Could you check a few things on this model? Use its own coordinates, in mm. Face numbers are marked on the shaded views. A direction names the side the tool comes from. Coordinates: 2 decimals unless noted, no trailing zeros. Order: outer loops, then holes, each group sorted by start corner. A loop starts at its lowest first (then second) coordinate and runs counter-clockwise, first axis right, second up.
```python
from build123d import *

# Parameters (mm, degrees)
F0_W     = 76.2
F0_H     = 36.11469
F1_DEPTH = 58.42
F0_R     = 12.858175
F2_DEPTH = 25.4
F3_R     = 6.059169
F4_DEPTH = 76.2
F5_DEPTH = 76.2
F7_DEPTH = 38.1


with BuildPart() as f1:
    # F0 (on Top) → F1 (new body)
    with BuildSketch(Plane.XY):
        Rectangle(F0_W, F0_H)
    extrude(amount=F1_DEPTH)

    # F0 (on Top) → F2 (join)
    with BuildSketch(Plane.XY):
        with BuildLine():
            Line((72.961012, 28.850658), (-72.961012, 28.850658))
            ThreePointArc((-72.961012, 28.850658), (-101.81167, 0), (-72.961012, -28.850658))
            Line((-72.961012, -28.850658), (72.961012, -28.850658))
            ThreePointArc((72.961012, -28.850658), (101.81167, 0), (72.961012, 28.850658))
        make_face()
        with Locations((-72.961012, 0)):
            Circle(F0_R, mode=Mode.SUBTRACT)
        Rectangle(F0_W, F0_H, mode=Mode.SUBTRACT)
        with Locations((72.961012, 0)):
            Circle(F0_R, mode=Mode.SUBTRACT)
    extrude(amount=F2_DEPTH)

    # F3 (on face) → F4 (join)
    with BuildSketch(Plane(origin=(-38.1, 0, 0), x_dir=(0, -1, 0), z_dir=(-1, 0, 0))):
        with Locations((0, 58.42)):
            Circle(F3_R)
        with BuildLine():
            Line((6.059169, 58.42), (18.057345, 58.42))
            ThreePointArc((18.057345, 58.42), (0, 76.477345), (-18.057345, 58.42))
            Line((-18.057345, 58.42), (-6.059169, 58.42))
            ThreePointArc((-6.059169, 58.42), (0, 64.479169), (6.059169, 58.42))
        make_face()
    extrude(amount=-F4_DEPTH)

    # F3 (on face) → F5 (cut)
    with BuildSketch(Plane(origin=(-38.1, 0, 0), x_dir=(0, -1, 0), z_dir=(-1, 0, 0))):
        with Locations((0, 58.42)):
            Circle(F3_R)
    extrude(amount=-F5_DEPTH, mode=Mode.SUBTRACT)

    # F6 (on Front) → F7 (cut, symmetric)
    with BuildSketch(Plane.XZ):
        with BuildLine():
            Line((16.832678, 103.529039), (-16.832678, 103.529039))
            Line((-16.832678, 103.529039), (-16.832678, 48.142973))
            ThreePointArc((-16.832678, 48.142973), (0, 31.310296), (16.832678, 48.142973))
            Line((16.832678, 48.142973), (16.832678, 103.529039))
        make_face()
    extrude(amount=F7_DEPTH, both=True, mode=Mode.SUBTRACT)


solid = f1.part
```
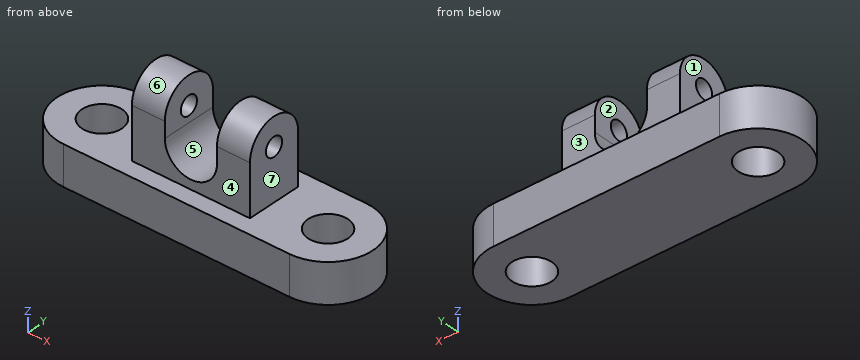
Item 1: Which directions (+Z, -Z, +X, -X, +Y, -Y) give clear straight access to the entire face, cutting with the end or side of a thin tool? Please do the marked faces 1, 2, 3 and 4.
Item 2: Thinking about a two-plate mould opening in X: for the marked faces 5, 6 and 7, which applies, +X half, -X half, draft (parallel to the pull), parting line (faces both ways), or undercut?
Item 3: I need wall thicknesses on line 1 (X direction, y = 1, z = 4.5); line 2 (Z direction, x = 33, y = 0); line 3 (X direction, y = 15.5, z = 56). Which ranges of each line are inside material? Lowest first, please.
Item 4: For pin 1 Ø18 at (y, z) = (-6, 44.5) entering from +X; pin 2 Ø4 at (x, y) = (-29, -17) entering from +Z; pin 3 Ø1.5 at (x, y) = (41, -22.5) entering from +Z, each with a flat end and sliding along its axis, tell me the tip position at first contact or that it passes through.
Item 5: Suppose I cut it at B-B (x = 33.5). List the corners of the cut face in (y, z) for me, and give its area (3 significant figures).
Item 6: Suppose I cut it at C-C (z = 36). List the corners of the cut face in (x, y) for me, and give its area (3 significant figures).
Item 7: Suppose I cut it at A-A (y = 0). List the corners of the cut face in (x, z) for me, and give its area (3 significant figures).
Item 8: Suppose I cut it at D-D (y = -9). List the corners of the cut face in (x, z) for me, and give its area (3 significant figures).
Geometry results:
1. face 1: +Z, -X, +Y, -Y
1. face 2: +Z, +Y, -Y
1. face 3: +Z, +X, -X, +Y
1. face 4: +Z, +X, -X, -Y
2. face 5: undercut
2. face 6: draft
2. face 7: +X half
3. line 1: x = -101.79 to -85.78, -60.14 to 60.14, 85.78 to 101.79
3. line 2: z = 0 to 52.36, 64.48 to 76.48
3. line 3: x = -38.1 to -16.83, 16.83 to 38.1
4. pin 1: stops at x = 38.1
4. pin 2: stops at z = 68.47
4. pin 3: stops at z = 25.4
5. outline: (-28.85, 0) - (28.85, 0) - (28.85, 25.4) - (18.06, 25.4) - (18.06, 58.42) arc R18.06 ccw to (-18.06, 58.42) - (-18.06, 25.4) - (-28.85, 25.4) - close; hole circle Ø12.12 at (0, 58.42)
5. area: 3,050 mm2
6. outline: (-38.1, -18.06) - (-11.66, -18.06) - (-11.66, 18.06) - (-38.1, 18.06) - close; (11.66, -18.06) - (38.1, -18.06) - (38.1, 18.06) - (11.66, 18.06) - close
6. area: 1,910 mm2
7. outline: (-101.81, 0) - (-85.82, 0) - (-85.82, 25.4) - (-101.81, 25.4) - close; (-60.1, 0) - (60.1, 0) - (60.1, 25.4) - (38.1, 25.4) - (38.1, 52.36) - (16.83, 52.36) - (16.83, 48.14) arc R16.83 cw to (-16.83, 48.14) - (-16.83, 52.36) - (-38.1, 52.36) - (-38.1, 25.4) - (-60.1, 25.4) - close; (-38.1, 64.48) - (-16.83, 64.48) - (-16.83, 76.48) - (-38.1, 76.48) - close; (16.83, 64.48) - (38.1, 64.48) - (38.1, 76.48) - (16.83, 76.48) - close; (85.82, 0) - (101.81, 0) - (101.81, 25.4) - (85.82, 25.4) - close
7. area: 5,840 mm2
8. outline: (-100.37, 0) - (-82.14, 0) - (-82.14, 25.4) - (-100.37, 25.4) - close; (-63.78, 0) - (63.78, 0) - (63.78, 25.4) - (38.1, 25.4) - (38.1, 74.07) - (16.83, 74.07) - (16.83, 48.14) arc R16.83 cw to (-16.83, 48.14) - (-16.83, 74.07) - (-38.1, 74.07) - (-38.1, 25.4) - (-63.78, 25.4) - close; (82.14, 0) - (100.37, 0) - (100.37, 25.4) - (82.14, 25.4) - close
8. area: 6,560 mm2
